Design review of the part built by this model. Coordinates are the model's own, in mm. Coordinates: 2 decimals unless noted, no trailing zeros. Write each loop counter-clockwise with the first axis right and the second up, starting at its lowest first coordinate (ties: lowest second). Pieces come first, ordered by that corner, then holes. Notation, with made-up numbers: (45.5, 70.25) -> (62.5, 70.25) arc R24 cw to (62.5, 102.25) -> close; hole circle Ø7 at (74.25, -28.75). An arc over 180 degrees is marked (long way). One line per question, with ' | ' between items. Start each with the question number.
Q1. Wall thickness on probe 1 along Z at (x, y) = (2, -2.25); probe 2 along X at (y, z) = (-1.5, -10.75); probe 3 along X at (y, z) = (-2, -10.5): over which ranges is each line inside the solid? List them lowest first.
Q2. Add section B-B on y = -5. State the section outline as (x, z) points, and give its area (3 significant figures).
Q3. Add section A-A on y = -1.5. State the section outline as (x, z) points, and give its area (3 significant figures).
Q4. For P1, Ø2, axis at x = 2.5, y = -0.5, coming from the -Z side; P2, Ø2, axis at x = -1.5, y = -3.5, coming from the -Z side, all flat-tipped, find the tip position at first contact; note any pin that passes through.
from build123d import *

# Parameters (mm, degrees)
F0_W     = 7
F0_H     = 25
F1_DEPTH = 5.5
F2_R     = 3
F3_R     = 1


with BuildPart() as f1:
    # F0 (on Front) → F1 (new body, symmetric)
    with BuildSketch(Plane.XZ):
        Rectangle(F0_W, F0_H)
    extrude(amount=F1_DEPTH, both=True)

    # F2
    f2_edges = [f1.edges().sort_by_distance(p)[0] for p in [
        (3.5, 0, 12.5),
        (-3.5, 0, 12.5),
        (3.5, 0, -12.5),
        (-3.5, 0, -12.5),
    ]]
    fillet(f2_edges, radius=F2_R)

    # F3
    f3_edges = [f1.edges().sort_by_distance(p)[0] for p in [
        (-3.5, -5.5, 0),
        (3.5, -5.5, 0),
        (-2.62132, -5.5, -11.62132),
        (2.62132, -5.5, 11.62132),
        (0, -5.5, -12.5),
        (-2.62132, -5.5, 11.62132),
        (0, -5.5, 12.5),
        (3.5, 5.5, 0),
        (-3.5, 5.5, 0),
        (0, 5.5, -12.5),
        (-2.62132, 5.5, -11.62132),
        (2.62132, 5.5, -11.62132),
        (-2.62132, 5.5, 11.62132),
        (2.62132, 5.5, 11.62132),
        (0, 5.5, 12.5),
    ]]
    fillet(f3_edges, radius=F3_R)


solid = f1.part
Output values:
1) probe 1: z = -12.1 to 12.1 | probe 2: x = -3.23 to 3.23 | probe 3: x = -3.33 to 3.33
2) outline: (-3.37, -9.5) arc R2.87 ccw to (-0.5, -12.37) -> (0.5, -12.37) arc R2.87 ccw to (3.37, -9.5) -> (3.37, 9.5) arc R2.87 ccw to (0.5, 12.37) -> (-0.5, 12.37) arc R2.87 ccw to (-3.37, 9.5) -> close | area: 159 mm2
3) outline: (-3.5, -9.5) arc R3 ccw to (-0.5, -12.5) -> (0.5, -12.5) arc R3 ccw to (3.5, -9.5) -> (3.5, 9.5) arc R3 ccw to (0.5, 12.5) -> (-0.5, 12.5) arc R3 ccw to (-3.5, 9.5) -> close | area: 167 mm2
4) P1: stops at z = -12.33 | P2: stops at z = -12.5
